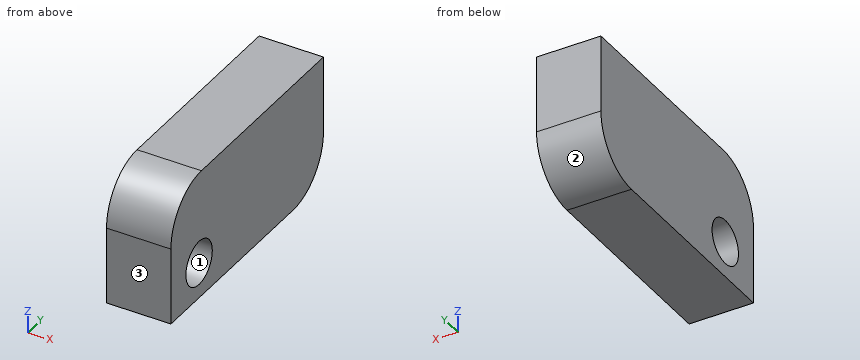
from build123d import *

# Parameters (mm, degrees)
F0_W     = 50.8
F0_H     = 25.4
F1_DEPTH = 12.7
F2_R     = 10.16
F3_R     = 4.389033
F4_DEPTH = 25.4


with BuildPart() as f1:
    # F0 (on Right) → F1 (new body)
    with BuildSketch(Plane.YZ):
        with Locations((25.4, -12.7)):
            Rectangle(F0_W, F0_H)
    extrude(amount=F1_DEPTH)

    # F2
    f2_edges = [f1.edges().sort_by_distance(p)[0] for p in [
        (6.35, 0, 0),
        (6.35, 50.8, -25.4),
    ]]
    fillet(f2_edges, radius=F2_R)

    # F3 (on face) → F4 (cut)
    with BuildSketch(Plane.YZ.offset(12.7)):
        with Locations((9.386016, -18.30278)):
            Circle(F3_R)
    extrude(amount=-F4_DEPTH, mode=Mode.SUBTRACT)


solid = f1.part
The listing builds one solid part. Answer for the finished solid, in the listing's coordinates (mm). Face numbers are marked on the shaded views. Give positions to 0.01 mm unless a question says otherwise; leave off trailing zeros. Write each loop counter-clockwise with the first axis right and the second up, starting at its lowest first coordinate (ties: lowest second). Pieces come first, ordered by that corner, then holes. Notation, with made-up numbers: (-19, 77.5) -> (-14, 77.5) arc R14 ccw to (-14, 97.5) -> close; hole circle Ø5 at (2, 29). An arc over 180 degrees is marked (long way). One line per question, with ' | ' between items. Start each with the question number.
1. For a pull along Z with two mould halves and no side action, classify the marked faces 1, 2 and 3 as pulls with the +Z half, pulls with the -Z half, needs draft (parallel to the pull), parting line crosses it, or undercut.
2. Given pin 1 Ø8 at (y, z) = (17.5, -21.5) entering from -X; pin 2 Ø7 at (y, z) = (9.39, -18.3) entering from +X, each flat-ended and moving along its own axis, determine where each tip first touches the part or whether it passes through.
3. Section A-A (z = -16.5) is taken. Determine the outline of the cut face in (x, y).
4. Section B-B (y = 12.5) is taken. Determine the outline of the cut face in (x, z), plus the area to 3 significant figures.
5. Section C-C (x = 6.75) is taken. Determine the outline of the cut face in (y, z).
6. Section D-D (z = -2.25) is taken. Determine the outline of the cut face in (x, y).
7. Find the intervals of material crossed by probe 1 along Z at (x, y) = (9.25, 6); probe 2 along Y at (x, z) = (11.5, -19.75); probe 3 along Y at (x, z) = (1.5, -20), in increasing order.
Response values:
1) face 1: undercut | face 2: pulls with the -Z half | face 3: needs draft
2) pin 1: x = 0 | pin 2: through
3) outline: (0, 0) -> (12.7, 0) -> (12.7, 5.38) -> (0, 5.38) -> close; (0, 13.39) -> (12.7, 13.39) -> (12.7, 50.72) -> (0, 50.72) -> close
4) outline: (0, -25.4) -> (12.7, -25.4) -> (12.7, -21.4) -> (0, -21.4) -> close; (0, -15.21) -> (12.7, -15.21) -> (12.7, 0) -> (0, 0) -> close | area: 244 mm2
5) outline: (0, -25.4) -> (40.64, -25.4) arc R10.16 ccw to (50.8, -15.24) -> (50.8, 0) -> (10.16, 0) arc R10.16 ccw to (0, -10.16) -> close; hole circle Ø8.78 at (9.39, -18.3)
6) outline: (0, 3.78) -> (12.7, 3.78) -> (12.7, 50.8) -> (0, 50.8) -> close
7) probe 1: -25.4 to -21.1, -15.51 to -0.89 | probe 2: 0 to 5.24, 13.53 to 49.74 | probe 3: 0 to 5.34, 13.43 to 49.62
